For this review, take the finished solid that the model builds, in its own axes (mm). Give positions to 0.01 mm unless a question says otherwise; leave off trailing zeros. Write each loop counter-clockwise with the first axis right and the second up, starting at its lowest first coordinate (ties: lowest second). Pieces come first, ordered by that corner, then holes.
from build123d import *

# Parameters (mm, degrees)
F1_DEPTH    = 5
F2_T1_DEPTH = 264.8076211353


# Not quite as in the source:
# - a fillet or chamfer that OpenCascade refuses, or shapes differently, is made with other operations: its cross-section is extruded or revolved along the edge and cut away or added


with BuildPart() as f1:
    # F0 (on Top) → F1 (new body)
    with BuildSketch(Plane.XY):
        Polygon((-0.6416016338, 191.2437425446), (-161.12652421, -89.6207541227), (162.3517262131, -88.1725256644), align=None)
    extrude(amount=F1_DEPTH)

    # F2: fillet of radius 30 on 3 edges, made by hand

    # F2_s2 → F2_t1 (cut)
    with BuildSketch(Plane.XY.offset(-129.9038105677)):
        with BuildLine():
            add(Edge.make_bspline(
                [(25.5403653575, 146.3605095453), (-0.6416016338, 191.2437425446), (-26.4206381195, 146.1278775095)],
                knots=[0, 0, 0, 1, 1, 1], degree=2, weights=[1, 1, 1]))
            Line((-26.4206381195, 146.1278775095), (-0.6416016338, 191.2437425446))
            Line((-0.6416016338, 191.2437425446), (25.5403653575, 146.3605095453))
        make_face()
        with BuildLine():
            add(Edge.make_bspline(
                [(-135.3474877243, -44.5048890876), (-161.12652421, -89.6207541227), (-109.165520733, -89.3881220869)],
                knots=[0, 0, 0, 1, 1, 1], degree=2, weights=[1, 1, 1]))
            Line((-109.165520733, -89.3881220869), (-161.12652421, -89.6207541227))
            Line((-161.12652421, -89.6207541227), (-135.3474877243, -44.5048890876))
        make_face()
        with BuildLine():
            add(Edge.make_bspline(
                [(136.1697592218, -43.2892926651), (162.3517262131, -88.1725256644), (110.3907227362, -88.4051577003)],
                knots=[0, 0, 0, 1, 1, 1], degree=2, weights=[1, 1, 1]))
            Line((110.3907227362, -88.4051577003), (162.3517262131, -88.1725256644))
            Line((162.3517262131, -88.1725256644), (136.1697592218, -43.2892926651))
        make_face()
    extrude(amount=F2_T1_DEPTH, mode=Mode.SUBTRACT)


solid = f1.part
(1) For L1, parallel to X at y = -49, z = 4.3; L2, parallel to X at y = 152, z = 2.35; L3, parallel to Y at x = 131.5, z = 4.1, list the stretches that pass through material, from the lowest coordinate up.
(2) We need section A-A (y = -2.5). Write out the cut boundary in (x, z).
(3) Clearance check with flat-ended pins moving along their axes: pin 1 Ø1.5 at (y, z) = (79, 1) entering from +X; pin 2 Ø1.5 at (y, z) = (26.5, 4.5) entering from +X. State where each tip first meets the part, or that it passes through.
(4) We need section B-B (x = 102). Write out the cut boundary in (y, z), and give its area (3 significant figures).
The answers:
1. L1: x = -137.78 to 139.28
1. L2: x = -22.81 to 22.01
1. L3: y = -85.49 to -35.28
2. outline: (-111.35, 0) - (112.38, 0) - (112.38, 5) - (-111.35, 5) - close
3. pin 1: stops at x = 65.27
3. pin 2: stops at x = 95.9
4. outline: (-88.44, 0) - (15.29, 0) - (15.29, 5) - (-88.44, 5) - close
4. area: 519 mm2
